Could you check a few things on this model? Use its own coordinates, in mm. A direction names the side the tool comes from. Coordinates: 2 decimals unless noted, no trailing zeros. Loops run counter-clockwise (first coordinate to the right, second up) from the corner with the lowest first, then second, coordinate; pieces in that order, holes last. Notation, with made-up numbers: (-5, 48) -> (43, 48) arc R14 cw to (43, 58) -> close; hole circle Ø1 at (0.5, 78.5). An arc over 180 degrees is marked (long way). One line per question, with ' | ' between items.
```python
from build123d import *

# Parameters (mm, degrees)
PAD_DEPTH       = 3
PAD001_DEPTH    = 40.3
SKETCH001_R     = 1.7
HOLE_DEPTH      = 3.001
SKETCH003_R     = 1.7
HOLE001_DEPTH   = 3.001
POCKET_DEPTH    = 3.001
POCKET001_DEPTH = 195.001
SKETCH008_W     = 53
SKETCH008_H     = 3
POCKET002_DEPTH = 40.301
SKETCH009_R     = 1.7
HOLE003_DEPTH   = 3.001
POCKET003_DEPTH = 5


with BuildPart() as part:
    # Sketch → Pad (new body)
    with BuildSketch(Plane.XY):
        Polygon((15, 39.748737), (39.748737, 15), (160.251263, 15), (185, 39.748737), (185, 170.251263), (160.251263, 195), (39.748737, 195), (15, 170.251263), align=None)
    extrude(amount=PAD_DEPTH)

    # Sketch002 → Pad001 (join)
    with BuildSketch(Plane.XY):
        Polygon((40, 194.944272), (48, 186), (152, 186), (160, 194.944272), align=None)
    extrude(amount=-PAD001_DEPTH)

    # Sketch001 → Hole (cut, through all)
    with BuildSketch(Plane.XY):
        with Locations((32.599303, 42.704115)):
            Circle(SKETCH001_R)
        with Locations((43.5, 32.4)):
            Circle(SKETCH001_R)
        with Locations((24, 37.6)):
            Circle(SKETCH001_R)
        with Locations((38.184146, 23.5)):
            Circle(SKETCH001_R)
        with Locations((161.184146, 23.5)):
            Circle(SKETCH001_R)
        with Locations((176.084785, 36.840575)):
            Circle(SKETCH001_R)
        with Locations((167.984236, 42.704115)):
            Circle(SKETCH001_R)
        with Locations((168.148156, 167.066578)):
            Circle(SKETCH001_R)
        with Locations((157.247459, 177.370693)):
            Circle(SKETCH001_R)
        with Locations((162.300682, 186)):
            Circle(SKETCH001_R)
        with Locations((176.748001, 172.16978)):
            Circle(SKETCH001_R)
        with Locations((32.599303, 166.895885)):
            Circle(SKETCH001_R)
        with Locations((43.33608, 177.370693)):
            Circle(SKETCH001_R)
        with Locations((38.282857, 186)):
            Circle(SKETCH001_R)
        with Locations((24, 172)):
            Circle(SKETCH001_R)
        with Locations((157.247459, 32.229307)):
            Circle(SKETCH001_R)
    extrude(amount=HOLE_DEPTH, mode=Mode.SUBTRACT)

    # Sketch003 → Hole001 (cut, through all)
    with BuildSketch(Plane.XY):
        with Locations((70, 160)):
            Circle(SKETCH003_R)
        with Locations((130, 160)):
            Circle(SKETCH003_R)
        with Locations((70, 50)):
            Circle(SKETCH003_R)
        with Locations((130, 50)):
            Circle(SKETCH003_R)
        with Locations((70, 105)):
            Circle(SKETCH003_R)
        with Locations((130, 123)):
            Circle(SKETCH003_R)
    extrude(amount=HOLE001_DEPTH, mode=Mode.SUBTRACT)

    # Sketch006 → Pocket (cut, through all)
    with BuildSketch(Plane.XY):
        with BuildLine():
            Line((65, 179.12132), (65, 167.12132))
            ThreePointArc((65, 167.12132), (65.62132, 165.62132), (67.12132, 165))
            Line((67.12132, 165), (132.87868, 165))
            ThreePointArc((132.87868, 165), (134.37868, 165.62132), (135, 167.12132))
            Line((135, 167.12132), (135, 179.12132))
            ThreePointArc((135, 179.12132), (134.37868, 180.62132), (132.87868, 181.242641))
            Line((132.87868, 181.242641), (67.12132, 181.242641))
            ThreePointArc((67.12132, 181.242641), (65.62132, 180.62132), (65, 179.12132))
        make_face()
        with BuildLine():
            Line((65, 39.12132), (65, 27.12132))
            ThreePointArc((65, 27.12132), (65.62132, 25.62132), (67.12132, 25))
            Line((67.12132, 25), (132.87868, 25))
            ThreePointArc((132.87868, 25), (134.37868, 25.62132), (135, 27.12132))
            Line((135, 27.12132), (135, 39.12132))
            ThreePointArc((135, 39.12132), (134.37868, 40.62132), (132.87868, 41.242641))
            Line((132.87868, 41.242641), (67.12132, 41.242641))
            ThreePointArc((67.12132, 41.242641), (65.62132, 40.62132), (65, 39.12132))
        make_face()
    extrude(amount=POCKET_DEPTH, mode=Mode.SUBTRACT)

    # Sketch007 → Pocket001 (cut, through all)
    with BuildSketch(Plane.XZ):
        with BuildLine():
            Line((75, -42), (125, -42))
            Line((125, -42), (125, -9.12132))
            ThreePointArc((125, -9.12132), (124.37868, -7.62132), (122.87868, -7))
            Line((122.87868, -7), (77.12132, -7))
            ThreePointArc((77.12132, -7), (75.62132, -7.62132), (75, -9.12132))
            Line((75, -9.12132), (75, -42))
        make_face()
    extrude(amount=-POCKET001_DEPTH, mode=Mode.SUBTRACT)

    # Sketch008 → Pocket002 (cut, through all)
    with BuildSketch(Plane.XY):
        with Locations((100, 191.5)):
            Rectangle(SKETCH008_W, SKETCH008_H)
    extrude(amount=-POCKET002_DEPTH, mode=Mode.SUBTRACT)

    # Sketch009 → Hole003 (cut, through all)
    with BuildSketch(Plane.XY):
        with Locations((50, 45)):
            Circle(SKETCH009_R)
        with Locations((150, 45)):
            Circle(SKETCH009_R)
        with Locations((150, 95)):
            Circle(SKETCH009_R)
        with Locations((50, 109)):
            Circle(SKETCH009_R)
        with Locations((50, 159)):
            Circle(SKETCH009_R)
        with Locations((150, 159)):
            Circle(SKETCH009_R)
    extrude(amount=HOLE003_DEPTH, mode=Mode.SUBTRACT)

    # Sketch010 → Pocket003 (cut)
    with BuildSketch(Plane.XY):
        Polygon((15, 55), (36.213203, 76.213203), (36.213203, 133.786797), (15, 155), align=None)
        Polygon((185, 55), (163.786797, 76.213203), (163.786797, 133.786797), (185, 155), align=None)
    extrude(amount=POCKET003_DEPTH, mode=Mode.SUBTRACT)


solid = part.part
```
Q1. Imagine slicing it at B-B on z = -13. Write out the boundary of the cut face in (x, y).
Values follow:
outline: (40, 194.94) -> (48, 186) -> (75, 186) -> (75, 190) -> (73.5, 190) -> (73.5, 193) -> (75, 193) -> (75, 194.94) -> close; (125, 186) -> (152, 186) -> (160, 194.94) -> (125, 194.94) -> (125, 193) -> (126.5, 193) -> (126.5, 190) -> (125, 190) -> close
Q2. For faces 1 (the face through (175, 65, 1)), 2 (the face through (155.944, 190.41, -19.868)), 3 (the face through (101.8, 193, -6.6)), 4 (the face through (99, 186, -6)), which set-ups out of +Z, -Z, +X, -X, +Y, -Y let a thin tool reach every point of the face, with its end or its side?
Values follow:
face 1: +Z, -Z, +X | face 2: -Z, +X, -Y | face 3: -Z | face 4: -Z, +X, -X, -Y
Q3. Imagine slicing it at A-A on x = 93. Write out the boundary of the cut face in (y, z), plus the area to 3 significant figures.
Values follow:
outline: (15, 0) -> (25, 0) -> (25, 3) -> (15, 3) -> close; (41.24, 0) -> (165, 0) -> (165, 3) -> (41.24, 3) -> close; (181.24, 0) -> (186, 0) -> (186, -7) -> (190, -7) -> (190, 0) -> (193, 0) -> (193, -7) -> (194.94, -7) -> (194.94, 0) -> (195, 0) -> (195, 3) -> (181.24, 3) -> close | area: 484 mm2
Q4. Imagine slicing it at D-D on y = 62.5. Write out the boundary of the cut face in (x, z).
Values follow:
outline: (22.5, 0) -> (177.5, 0) -> (177.5, 3) -> (22.5, 3) -> close
Q5. For pin 1 (1.6 mm diameter, centred on y = 194, z = -29.5, fed in from -X); pin 2 (2.5 mm diameter, centred on x = 24, y = 172, fed in from +Z); pin 3 (4.5 mm diameter, centred on x = 157.25, y = 32.23, fed in from -Z); pin 4 (1.6 mm diameter, centred on x = 96.5, y = 194.5, fed in from -Z), each with a flat end and sliding along its axis, tell me the tip position at first contact or that it passes through.
Values follow:
pin 1: stops at x = 40.13 | pin 2: passes through | pin 3: stops at z = 0 | pin 4: stops at z = -7
Q6. Please list where these lines run through material, in increasing order: L1, parallel to Y at x = 130, z = 0.95; L2, parallel to X at y = 45, z = 1.7; L3, parallel to X at y = 160, z = 2.15. Write a range as [from, to].
Values follow:
L1: y = [15, 25], [41.24, 48.3], [51.7, 121.3], [124.7, 158.3], [161.7, 165], [181.24, 195] | L2: x = [15, 48.3], [51.7, 148.3], [151.7, 185] | L3: x = [15, 48.63], [51.37, 68.3], [71.7, 128.3], [131.7, 148.63], [151.37, 185]
Q7. We'd pull the mould along Y, two halves only. Please class faces 5 (the face through (43.944, 190.535, -19.868)), 6 (the face through (75, 188, -24)), 7 (the face through (25, 65, 1)): released by +Y, released by -Y, zero draft, split by the parting line, or undercut.
Values follow:
face 5: released by -Y | face 6: zero draft | face 7: undercut
Q8. Imagine slicing it at C-C on z = -3.5. Write out the boundary of the cut face in (x, y), plus the area to 3 significant figures.
Values follow:
outline: (40, 194.94) -> (48, 186) -> (152, 186) -> (160, 194.94) -> close; hole (73.5, 190) -> (126.5, 190) -> (126.5, 193) -> (73.5, 193) -> close | area: 843 mm2
